The model under review builds one solid part; all positions refer to its coordinate system, in mm. A direction names the side the tool comes from. Give positions to 0.01 mm unless a question says otherwise; leave off trailing zeros. Order: outer loops, then holes, each group sorted by start corner. A loop starts at its lowest first (then second) coordinate and runs counter-clockwise, first axis right, second up. Notation, with made-up numbers: (-20, -25) - (36, -25) arc R12 cw to (36, -14) - close; hole circle Ø5 at (-17.5, 86). An arc over 180 degrees is marked (long way). Put each result on its own line as item: value.
```python
from build123d import *

# Parameters (mm, degrees)
SKETCH_1_R      = 1.4
EXTRUDE_1_DEPTH = 15
SKETCH_2_R      = 1.682017604
EXTRUDE_2_DEPTH = 10
EXTRUDE_3_DEPTH = 2
SKETCH_4_W      = 8.385315984
SKETCH_4_H      = 7.611286816
SKETCH_4_W_2    = 5.805218758
SKETCH_4_H_2    = 5.031189591
SKETCH_4_W_3    = 6.708252787
SKETCH_4_H_3    = 5.869721189
SKETCH_4_W_4    = 19.737743777
SKETCH_4_H_4    = 3.483131255
EXTRUDE_4_DEPTH = 1


with BuildPart() as part:
    # 草图1 → 凸台-拉伸1 (new body)
    with BuildSketch(Plane(origin=(0, 0, 0), x_dir=(1, 0, 0), z_dir=(0, 1, 0))):
        Polygon((80, 53), (80, 0), (0, 0), (0, 53), (39.5, 53), (41.5, 53), align=None)
        with Locations((76, 50.5)):
            Circle(SKETCH_1_R, mode=Mode.SUBTRACT)
        with Locations((76, 2.5)):
            Circle(SKETCH_1_R, mode=Mode.SUBTRACT)
        with Locations((4, 50.5)):
            Circle(SKETCH_1_R, mode=Mode.SUBTRACT)
        with Locations((4, 2.5)):
            Circle(SKETCH_1_R, mode=Mode.SUBTRACT)
    extrude(amount=EXTRUDE_1_DEPTH)

    # 草图2 → 凸台-拉伸2 (add)
    with BuildSketch(Plane(origin=(0, 15, 0), x_dir=(1, 0, 0), z_dir=(0, 1, 0))):
        with Locations((10.586891626, 47.721299682)):
            Circle(SKETCH_2_R)
        with Locations((15.586891626, 47.721299682)):
            Circle(SKETCH_2_R)
        with Locations((20.586891626, 47.721299682)):
            Circle(SKETCH_2_R)
        with Locations((25.586891626, 47.721299682)):
            Circle(SKETCH_2_R)
        with Locations((30.586891626, 47.721299682)):
            Circle(SKETCH_2_R)
        with Locations((35.586891626, 47.721299682)):
            Circle(SKETCH_2_R)
        with Locations((40.586891626, 47.721299682)):
            Circle(SKETCH_2_R)
        with Locations((45.586891626, 47.721299682)):
            Circle(SKETCH_2_R)
        with Locations((50.586891626, 47.721299682)):
            Circle(SKETCH_2_R)
        with Locations((55.586891626, 47.721299682)):
            Circle(SKETCH_2_R)
        with Locations((60.586891626, 47.721299682)):
            Circle(SKETCH_2_R)
        with Locations((65.586891626, 47.721299682)):
            Circle(SKETCH_2_R)
        with Locations((70.586891626, 47.721299682)):
            Circle(SKETCH_2_R)
        with Locations((15.586891626, 42.721299682)):
            Circle(SKETCH_2_R)
        with Locations((20.586891626, 42.721299682)):
            Circle(SKETCH_2_R)
        with Locations((25.586891626, 42.721299682)):
            Circle(SKETCH_2_R)
        with Locations((30.586891626, 42.721299682)):
            Circle(SKETCH_2_R)
        with Locations((35.586891626, 42.721299682)):
            Circle(SKETCH_2_R)
        with Locations((40.586891626, 42.721299682)):
            Circle(SKETCH_2_R)
        with Locations((45.586891626, 42.721299682)):
            Circle(SKETCH_2_R)
        with Locations((50.586891626, 42.721299682)):
            Circle(SKETCH_2_R)
        with Locations((55.586891626, 42.721299682)):
            Circle(SKETCH_2_R)
        with Locations((60.586891626, 42.721299682)):
            Circle(SKETCH_2_R)
        with Locations((65.586891626, 42.721299682)):
            Circle(SKETCH_2_R)
        with Locations((70.586891626, 42.721299682)):
            Circle(SKETCH_2_R)
        with Locations((15.586891626, 37.721299682)):
            Circle(SKETCH_2_R)
        with Locations((20.586891626, 37.721299682)):
            Circle(SKETCH_2_R)
        with Locations((25.586891626, 37.721299682)):
            Circle(SKETCH_2_R)
        with Locations((30.586891626, 37.721299682)):
            Circle(SKETCH_2_R)
        with Locations((35.586891626, 37.721299682)):
            Circle(SKETCH_2_R)
        with Locations((40.586891626, 37.721299682)):
            Circle(SKETCH_2_R)
        with Locations((45.586891626, 37.721299682)):
            Circle(SKETCH_2_R)
        with Locations((50.586891626, 37.721299682)):
            Circle(SKETCH_2_R)
        with Locations((55.586891626, 37.721299682)):
            Circle(SKETCH_2_R)
        with Locations((60.586891626, 37.721299682)):
            Circle(SKETCH_2_R)
        with Locations((65.586891626, 37.721299682)):
            Circle(SKETCH_2_R)
        with Locations((70.586891626, 37.721299682)):
            Circle(SKETCH_2_R)
        with Locations((10.586891626, 42.721299682)):
            Circle(SKETCH_2_R)
        with Locations((10.586891626, 37.721299682)):
            Circle(SKETCH_2_R)
    extrude(amount=EXTRUDE_2_DEPTH)

    # 草图3 → 凸台-拉伸3 (add)
    with BuildSketch(Plane(origin=(0, 15, 0), x_dir=(1, 0, 0), z_dir=(0, 1, 0))):
        with BuildLine():
            Line((20.586891626, 27.53161424), (20.586891626, 13.083919076))
            ThreePointArc((20.586891626, 13.083919076), (21.172678064, 11.669705513), (22.586891626, 11.083919076))
            Line((22.586891626, 11.083919076), (24.521115245, 11.083919076))
            ThreePointArc((24.521115245, 11.083919076), (25.935328808, 11.669705513), (26.521115245, 13.083919076))
            Line((26.521115245, 13.083919076), (26.521115245, 27.53161424))
            ThreePointArc((26.521115245, 27.53161424), (25.935328808, 28.945827803), (24.521115245, 29.53161424))
            Line((24.521115245, 29.53161424), (22.586891626, 29.53161424))
            ThreePointArc((22.586891626, 29.53161424), (21.172678064, 28.945827803), (20.586891626, 27.53161424))
        make_face()
        with BuildLine():
            Line((12.586891626, 29.53161424), (14.521115245, 29.53161424))
            ThreePointArc((14.521115245, 29.53161424), (15.935328808, 28.945827803), (16.521115245, 27.53161424))
            Line((16.521115245, 27.53161424), (16.521115245, 13.083919076))
            ThreePointArc((16.521115245, 13.083919076), (15.935328808, 11.669705513), (14.521115245, 11.083919076))
            Line((14.521115245, 11.083919076), (12.586891626, 11.083919076))
            ThreePointArc((12.586891626, 11.083919076), (11.172678064, 11.669705513), (10.586891626, 13.083919076))
            Line((10.586891626, 13.083919076), (10.586891626, 27.53161424))
            ThreePointArc((10.586891626, 27.53161424), (11.172678064, 28.945827803), (12.586891626, 29.53161424))
        make_face()
        with BuildLine():
            Line((30.586891626, 27.53161424), (30.586891626, 13.083919076))
            ThreePointArc((30.586891626, 13.083919076), (31.172678064, 11.669705513), (32.586891626, 11.083919076))
            Line((32.586891626, 11.083919076), (34.521115245, 11.083919076))
            ThreePointArc((34.521115245, 11.083919076), (35.935328808, 11.669705513), (36.521115245, 13.083919076))
            Line((36.521115245, 13.083919076), (36.521115245, 27.53161424))
            ThreePointArc((36.521115245, 27.53161424), (35.935328808, 28.945827803), (34.521115245, 29.53161424))
            Line((34.521115245, 29.53161424), (32.586891626, 29.53161424))
            ThreePointArc((32.586891626, 29.53161424), (31.172678064, 28.945827803), (30.586891626, 27.53161424))
        make_face()
        with BuildLine():
            Line((40.586891626, 27.53161424), (40.586891626, 13.083919076))
            ThreePointArc((40.586891626, 13.083919076), (41.172678064, 11.669705513), (42.586891626, 11.083919076))
            Line((42.586891626, 11.083919076), (44.521115245, 11.083919076))
            ThreePointArc((44.521115245, 11.083919076), (45.935328808, 11.669705513), (46.521115245, 13.083919076))
            Line((46.521115245, 13.083919076), (46.521115245, 27.53161424))
            ThreePointArc((46.521115245, 27.53161424), (45.935328808, 28.945827803), (44.521115245, 29.53161424))
            Line((44.521115245, 29.53161424), (42.586891626, 29.53161424))
            ThreePointArc((42.586891626, 29.53161424), (41.172678064, 28.945827803), (40.586891626, 27.53161424))
        make_face()
    extrude(amount=EXTRUDE_3_DEPTH)

    # 草图4 → 凸台-拉伸4 (add)
    with BuildSketch(Plane(origin=(0, 15, 0), x_dir=(1, 0, 0), z_dir=(0, 1, 0))):
        with Locations((61.479309405, 26.5)):
            Rectangle(SKETCH_4_W, SKETCH_4_H)
        with Locations((56.190110092, 14.244538178)):
            Rectangle(SKETCH_4_W_2, SKETCH_4_H_2)
        with Locations((68.252064623, 17.179398772)):
            Rectangle(SKETCH_4_W_3, SKETCH_4_H_3)
        with Locations((61.737319128, 6.246236778)):
            Rectangle(SKETCH_4_W_4, SKETCH_4_H_4)
    extrude(amount=EXTRUDE_4_DEPTH)


solid = part.part
```
(1) The part is to be moulded in two halves that separate along X. For faces 1 (the flat face through (80, 7, -27)), 2 (the cylindrical face through (21.363, 19.93, -36.229)), 3 (the cylindrical face through (9.25, 19.93, -36.7)), 4 (the flat face through (56, 25, -48)), say which applies: pulls with the +X half, pulls with the -X half, needs draft (parallel to the pull), parting line crosses it, or undercut.
The answers:
face 1: pulls with the +X half
face 2: undercut
face 3: undercut
face 4: needs draft
(2) Take a section at B-B, the plane x = 76. Write out the cut boundary in (y, z).
The answers:
outline: (0, -53) - (15, -53) - (15, -51.9) - (0, -51.9) - close; (0, -49.1) - (15, -49.1) - (15, -3.9) - (0, -3.9) - close; (0, -1.1) - (15, -1.1) - (15, 0) - (0, 0) - close
(3) For faces 5 (the flat face through (14, 16, -29.532)), 6 (the flat face through (0, 7, -26)), 7 (the flat face through (44, 16, -11.084)), 8 (the flat face through (16, 25, -48)), 9 (the cylindrical face through (26.363, 19.93, -41.229)), list the 3-axis set-ups (+Z, -Z, +X, -X, +Y, -Y) from which the entire face can be reached by the end or side of a thin tool; tool diameter is ignored.
The answers:
face 5: -X, +Y
face 6: +Z, -Z, -X, +Y, -Y
face 7: +Z, +X, -X, +Y
face 8: +Z, -Z, +X, -X, +Y
face 9: +Y
(4) Wall thickness on L1, parallel to X at y = 9, z = -50.5; L2, parallel to Z at x = 4, y = 10.25; L3, parallel to Z at x = 42, y = 22.25: over which ranges is each line inside the solid? List them lowest first.
The answers:
L1: 0 to 2.6, 5.4 to 74.6, 77.4 to 80
L2: -53 to -51.9, -49.1 to -3.9, -1.1 to 0
L3: -48.63 to -46.81, -43.63 to -41.81, -38.63 to -36.81
(5) Clearance check with flat-ended pins moving along their axes: pin 1 Ø0.6 at (y, z) = (15.5, -19) entering from +X; pin 2 Ø8.5 at (x, z) = (59.5, -24.5) entering from +Y; pin 3 Ø0.5 at (y, z) = (15.5, -25.5) entering from -X. State where each tip first meets the part, or that it passes through.
The answers:
pin 1: x = 71.61
pin 2: y = 16
pin 3: x = 10.59
(6) Take a section at A-A, the plane z = -50.5. Write out the cut boundary in (x, y).
The answers:
outline: (0, 0) - (2.6, 0) - (2.6, 15) - (0, 15) - close; (5.4, 0) - (74.6, 0) - (74.6, 15) - (5.4, 15) - close; (77.4, 0) - (80, 0) - (80, 15) - (77.4, 15) - close
